```python
from build123d import *

# Parameters (mm, degrees)
SKETCH1_R                                  = 19
BODY_DEPTH                                 = 3
SPRING_PROFILE_DEPTH                       = 3
SPRING_PATTERN_COUNT                       = 2
SPRING_PATTERN_PITCH                       = 6
SKETCH5_W                                  = 2.5
SKETCH5_H                                  = 3
SPRING_EXTENSION_DEPTH                     = 1
MIRROR1_COPY_1_DEPTH                       = 3
MIRROR1_AT_THE_SECOND_PLANE_COPY_1_DEPTH   = 3
MIRROR1_AT_THE_SECOND_PLANE_COPY_2_DEPTH   = 3
MIRROR1_AT_THE_SECOND_PLANE_COPY_3_SKETC_W = 2.5
MIRROR1_AT_THE_SECOND_PLANE_COPY_3_SKETC_H = 3
MIRROR1_AT_THE_SECOND_PLANE_COPY_3_DEPTH   = 1
MIRROR1_AT_THE_SECOND_PLANE_COPY_4_DEPTH   = 3
CLAMP_DEPTH                                = 3.25
SKETCH6_R                                  = 1.6
SCREW_HOLES_DEPTH                          = 46.364202575
SCREW_CHAMFER_SIZE                         = 2


with BuildPart() as part:
    # Sketch1 → Body (new body)
    with BuildSketch(Plane(origin=(0, 0, 0), x_dir=(1, 0, 0), z_dir=(0, 1, 0))):
        with Locations(Location((0, 0, 0), (0, 0, 270))):
            Circle(SKETCH1_R)
    extrude(amount=BODY_DEPTH)

    # Sketch2 → Spring profile (add)
    with BuildSketch(Plane(origin=(0, 0, 0), x_dir=(1, 0, 0), z_dir=(0, 1, 0))):
        with BuildLine():
            ThreePointArc((3.25, 16.5), (3.323223305, 16.676776695), (3.5, 16.75))
            Line((3.5, 16.75), (8.5, 16.75))
            ThreePointArc((8.5, 16.75), (11.25, 19.5), (8.5, 22.25))
            Line((8.5, 22.25), (3.5, 22.25))
            ThreePointArc((3.5, 22.25), (3.323223305, 22.323223305), (3.25, 22.5))
            Line((3.25, 22.5), (0.75, 22.5))
            ThreePointArc((0.75, 22.5), (1.555456352, 20.555456352), (3.5, 19.75))
            Line((3.5, 19.75), (8.5, 19.75))
            ThreePointArc((8.5, 19.75), (8.75, 19.5), (8.5, 19.25))
            Line((8.5, 19.25), (3.5, 19.25))
            ThreePointArc((3.5, 19.25), (1.555456352, 18.444543648), (0.75, 16.5))
            Line((0.75, 16.5), (3.25, 16.5))
        make_face()
    spring_profile = extrude(amount=SPRING_PROFILE_DEPTH)

    # Spring pattern: Spring profile ×2
    with Locations(*[(0, 0, -i * SPRING_PATTERN_PITCH) for i in range(1, SPRING_PATTERN_COUNT)]):
        add(spring_profile)

    # Sketch5 → Spring extension (add)
    with BuildSketch(Plane(origin=(0, 0, -28.5), x_dir=(-1, 0, 0), z_dir=(0, 0, -1))):
        with Locations((-2, 1.5)):
            Rectangle(SKETCH5_W, SKETCH5_H)
    spring_extension = extrude(amount=SPRING_EXTENSION_DEPTH)

    # Mirror1: Spring profile, Spring extension across plane
    add(spring_profile.mirror(Plane.XY))
    add(spring_extension.mirror(Plane.XY))

    # Mirror1 copy 1 sketch → Mirror1 copy 1 (add)
    with BuildSketch(Plane(origin=(0, 0, 6), x_dir=(1, 0, 0), z_dir=(0, 1, 0))):
        with BuildLine():
            ThreePointArc((3.25, -16.5), (3.323223305, -16.676776695), (3.5, -16.75))
            Line((3.5, -16.75), (8.5, -16.75))
            ThreePointArc((8.5, -16.75), (11.25, -19.5), (8.5, -22.25))
            Line((8.5, -22.25), (3.5, -22.25))
            ThreePointArc((3.5, -22.25), (3.323223305, -22.323223305), (3.25, -22.5))
            Line((3.25, -22.5), (0.75, -22.5))
            ThreePointArc((0.75, -22.5), (1.555456352, -20.555456352), (3.5, -19.75))
            Line((3.5, -19.75), (8.5, -19.75))
            ThreePointArc((8.5, -19.75), (8.75, -19.5), (8.5, -19.25))
            Line((8.5, -19.25), (3.5, -19.25))
            ThreePointArc((3.5, -19.25), (1.555456352, -18.444543648), (0.75, -16.5))
            Line((0.75, -16.5), (3.25, -16.5))
        make_face()
    extrude(amount=MIRROR1_COPY_1_DEPTH)

    # Mirror1 at the second plane: Spring profile, Spring extension across plane
    add(spring_profile.mirror(Plane(origin=(0, 0, 0), x_dir=(0, 0, 1), z_dir=(1, 0, 0))))
    add(spring_extension.mirror(Plane(origin=(0, 0, 0), x_dir=(0, 0, 1), z_dir=(1, 0, 0))))

    # Mirror1 at the second plane copy 1 sketc → Mirror1 at the second plane copy 1 (add)
    with BuildSketch(Plane(origin=(0, 0, -6), x_dir=(-1, 0, 0), z_dir=(0, 1, 0))):
        with BuildLine():
            ThreePointArc((3.25, -16.5), (3.323223305, -16.676776695), (3.5, -16.75))
            Line((3.5, -16.75), (8.5, -16.75))
            ThreePointArc((8.5, -16.75), (11.25, -19.5), (8.5, -22.25))
            Line((8.5, -22.25), (3.5, -22.25))
            ThreePointArc((3.5, -22.25), (3.323223305, -22.323223305), (3.25, -22.5))
            Line((3.25, -22.5), (0.75, -22.5))
            ThreePointArc((0.75, -22.5), (1.555456352, -20.555456352), (3.5, -19.75))
            Line((3.5, -19.75), (8.5, -19.75))
            ThreePointArc((8.5, -19.75), (8.75, -19.5), (8.5, -19.25))
            Line((8.5, -19.25), (3.5, -19.25))
            ThreePointArc((3.5, -19.25), (1.555456352, -18.444543648), (0.75, -16.5))
            Line((0.75, -16.5), (3.25, -16.5))
        make_face()
    extrude(amount=MIRROR1_AT_THE_SECOND_PLANE_COPY_1_DEPTH)

    # Mirror1 at the second plane copy 2 sketc → Mirror1 at the second plane copy 2 (add)
    with BuildSketch(Plane(origin=(0, 0, 0), x_dir=(-1, 0, 0), z_dir=(0, 1, 0))):
        with BuildLine():
            ThreePointArc((3.25, 16.5), (3.323223305, 16.676776695), (3.5, 16.75))
            Line((3.5, 16.75), (8.5, 16.75))
            ThreePointArc((8.5, 16.75), (11.25, 19.5), (8.5, 22.25))
            Line((8.5, 22.25), (3.5, 22.25))
            ThreePointArc((3.5, 22.25), (3.323223305, 22.323223305), (3.25, 22.5))
            Line((3.25, 22.5), (0.75, 22.5))
            ThreePointArc((0.75, 22.5), (1.555456352, 20.555456352), (3.5, 19.75))
            Line((3.5, 19.75), (8.5, 19.75))
            ThreePointArc((8.5, 19.75), (8.75, 19.5), (8.5, 19.25))
            Line((8.5, 19.25), (3.5, 19.25))
            ThreePointArc((3.5, 19.25), (1.555456352, 18.444543648), (0.75, 16.5))
            Line((0.75, 16.5), (3.25, 16.5))
        make_face()
    extrude(amount=MIRROR1_AT_THE_SECOND_PLANE_COPY_2_DEPTH)



with BuildPart() as body_2:
    # Mirror1 at the second plane copy 3 sketc → Mirror1 at the second plane copy 3 (new body)
    with BuildSketch(Plane.XY.offset(28.5)):
        with Locations((-2, 1.5)):
            Rectangle(MIRROR1_AT_THE_SECOND_PLANE_COPY_3_SKETC_W, MIRROR1_AT_THE_SECOND_PLANE_COPY_3_SKETC_H)
    extrude(amount=MIRROR1_AT_THE_SECOND_PLANE_COPY_3_DEPTH)


with BuildPart() as part_1:
    add(part.part)

    add(body_2.part)  # Mirror1 at the second plane copy 4 merges body 2
    # Mirror1 at the second plane copy 4 sketc → Mirror1 at the second plane copy 4 (add)
    with BuildSketch(Plane(origin=(0, 0, 6), x_dir=(-1, 0, 0), z_dir=(0, 1, 0))):
        with BuildLine():
            ThreePointArc((3.25, 16.5), (3.323223305, 16.676776695), (3.5, 16.75))
            Line((3.5, 16.75), (8.5, 16.75))
            ThreePointArc((8.5, 16.75), (11.25, 19.5), (8.5, 22.25))
            Line((8.5, 22.25), (3.5, 22.25))
            ThreePointArc((3.5, 22.25), (3.323223305, 22.323223305), (3.25, 22.5))
            Line((3.25, 22.5), (0.75, 22.5))
            ThreePointArc((0.75, 22.5), (1.555456352, 20.555456352), (3.5, 19.75))
            Line((3.5, 19.75), (8.5, 19.75))
            ThreePointArc((8.5, 19.75), (8.75, 19.5), (8.5, 19.25))
            Line((8.5, 19.25), (3.5, 19.25))
            ThreePointArc((3.5, 19.25), (1.555456352, 18.444543648), (0.75, 16.5))
            Line((0.75, 16.5), (3.25, 16.5))
        make_face()
    extrude(amount=MIRROR1_AT_THE_SECOND_PLANE_COPY_4_DEPTH)

    # Sketch4 → Clamp (add, symmetric)
    with BuildSketch(Plane(origin=(0, 0, 0), x_dir=(0, 0, -1), z_dir=(1, 0, 0))):
        with BuildLine():
            Line((32, 0), (29.5, 0))
            Line((29.5, 0), (29.5, 3))
            Line((29.5, 3), (32, 3))
            ThreePointArc((32, 3), (35.863703305, 5.96472382), (34, 10.464101615))
            ThreePointArc((34, 10.464101615), (33.450961894, 12.513139721), (35.5, 13.062177826))
            ThreePointArc((35.5, 13.062177826), (38.761480784, 5.188266684), (32, 0))
        make_face()
    clamp = extrude(amount=CLAMP_DEPTH, both=True)

    # Mirror2: Clamp across plane
    add(clamp.mirror(Plane.XY))

    # Sketch6 → Screw holes (cut, through all)
    with BuildSketch(Plane(origin=(0, 0, 0), x_dir=(1, 0, 0), z_dir=(0, 1, 0))):
        with Locations(Location((0, -8, 0), (0, 0, 270))):
            Circle(SKETCH6_R)
        with Locations(Location((0, 8, 0), (0, 0, 270))):
            Circle(SKETCH6_R)
    extrude(amount=SCREW_HOLES_DEPTH, mode=Mode.SUBTRACT)

    # Screw chamfer
    screw_chamfer_edges = [part_1.edges().sort_by_distance(p)[0] for p in [
        (0, 3, 6.4),
        (0, 3, -9.6),
    ]]
    chamfer(screw_chamfer_edges, length=SCREW_CHAMFER_SIZE)


solid = part_1.part
```
Model file for the job. Use its own axes, mm. A direction names the side the tool comes from. Round coordinates to 2 decimals unless told otherwise and drop trailing zeros. Write each loop counter-clockwise with the first axis right and the second up, starting at its lowest first coordinate (ties: lowest second). Pieces come first, ordered by that corner, then holes. Notation, with made-up numbers: (76.5, 78) - (91.5, 78) arc R18 cw to (91.5, 109) - close; hole circle Ø9 at (14.25, 74.5). An arc over 180 degrees is marked (long way). Use CSV: the item, a comma, the result in double quotes. Start each with the question number.
Item 1: Pin check, flat tips, straight feed: P1, Ø3.5, axis at x = -7, y = 1, coming from the +Z side; P2, Ø3, axis at x = -4.5, z = -16.5, coming from the +Y side; P3, Ø2.5, axis at x = -6, y = 1, coming from the -Z side; P4, Ø4, axis at x = 13, z = 23.5, coming from the -Y side. Stop position of each tip, or through.
Item 2: Two-plate mould, pull along X, no slides. Class faces 1 (the face through (-11.25, 1.48, 25.44)), 2 (the face through (0.046, 12.484, 33.435)), 3 (the face through (2.8, 1.48, -19.16)): released by +X, released by -X, zero draft, split by the parting line, or undercut.
Item 3: Drill centre lines: L1, parallel to Z at x = -1, y = 7.25; L2, parallel to X at y = 2, z = -35; L3, parallel to Y at x = 2, z = -21.5. Where is each one in solid material? Low to high. Write a range as [from, to].
Item 4: Band-saw the part on B-B (y = 7). Write the cut outline in (x, z).
Item 5: Band-saw the part on D-D (z = 34.75). Write the cut outline in (x, y), and give its area (3 significant figures).
Item 6: Tool access for faces 4 (the face through (-6, 1, 19.25)), 5 (the face through (6, 1, -22.25)), 6 (the face through (-3.25, 5, -36)): list every direction of +Z, -Z, +X, -X, +Y, -Y with a clear straight run to the whole face (end or side of a thin tool).
Item 7: Band-saw the part on C-C (x = 0). Write the cut outline in (y, z).
Item 8: Band-saw the part on A-A (x = 6). Write the cut outline in (y, z), and give its area (4 significant figures).
Checked values:
1,P1,"stops at z = 28.25"
1,P2,"stops at y = 3"
1,P3,"stops at z = -28.25"
1,P4,"passes through"
2,face 1,"released by -X"
2,face 2,"zero draft"
2,face 3,"undercut"
3,L1,"z = [-39, -35.99], [35.99, 39]"
3,L2,"x = [-3.25, 3.25]"
3,L3,"y = [0, 3]"
4,outline,"(-3.25, -39) - (3.25, -39) - (3.25, -36) - (-3.25, -36) - close; (-3.25, 36) - (3.25, 36) - (3.25, 39) - (-3.25, 39) - close"
5,outline,"(-3.25, 0.56) - (3.25, 0.56) - (3.25, 4.1) - (-3.25, 4.1) - close; (-3.25, 9.9) - (3.25, 9.9) - (3.25, 13.26) - (-3.25, 13.26) - close"
5,area,"44.8 mm²"
6,face 4,"+Y, -Y"
6,face 5,"+X, +Y, -Y"
6,face 6,"-Z, -X, +Y, -Y"
7,outline,"(0, -32) arc R7 ccw to (13.06, -35.5) arc R1.5 ccw to (10.46, -34) arc R4 cw to (3, -32) - (3, -29.5) - (0, -29.5) - close; (0, -19) - (3, -19) - (3, -11.6) - (1, -9.6) - (0, -9.6) - close; (0, -6.4) - (1, -6.4) - (3, -4.4) - (3, 4.4) - (1, 6.4) - (0, 6.4) - close; (0, 9.6) - (1, 9.6) - (3, 11.6) - (3, 19) - (0, 19) - close; (0, 29.5) - (3, 29.5) - (3, 32) arc R4 cw to (10.46, 34) arc R1.5 ccw to (13.06, 35.5) arc R7 ccw to (0, 32) - close"
8,outline,"(0, -28.25) - (3, -28.25) - (3, -25.75) - (0, -25.75) - close; (0, -25.25) - (3, -25.25) - (3, -22.75) - (0, -22.75) - close; (0, -22.25) - (3, -22.25) - (3, -19.75) - (0, -19.75) - close; (0, -19.25) - (3, -19.25) - (3, 19.25) - (0, 19.25) - close; (0, 19.75) - (3, 19.75) - (3, 22.25) - (0, 22.25) - close; (0, 22.75) - (3, 22.75) - (3, 25.25) - (0, 25.25) - close; (0, 25.75) - (3, 25.75) - (3, 28.25) - (0, 28.25) - close"
8,area,"160.5 mm²"
